For this review, use the dimensioned drawing (mm, ordinates from the lowest corner) and the shaded views. A direction names the side the tool comes from. Coordinates: 2 decimals unless noted, no trailing zeros. Loops run counter-clockwise (first coordinate to the right, second up) from the corner with the lowest first, then second, coordinate; pieces in that order, holes last. Notation, with made-up numbers: M 8,44 L 46,44 A13 cw 46,55 Z; hole C -20,70 d2. An arc over 180 degrees is marked long. One line per item, written item: value.
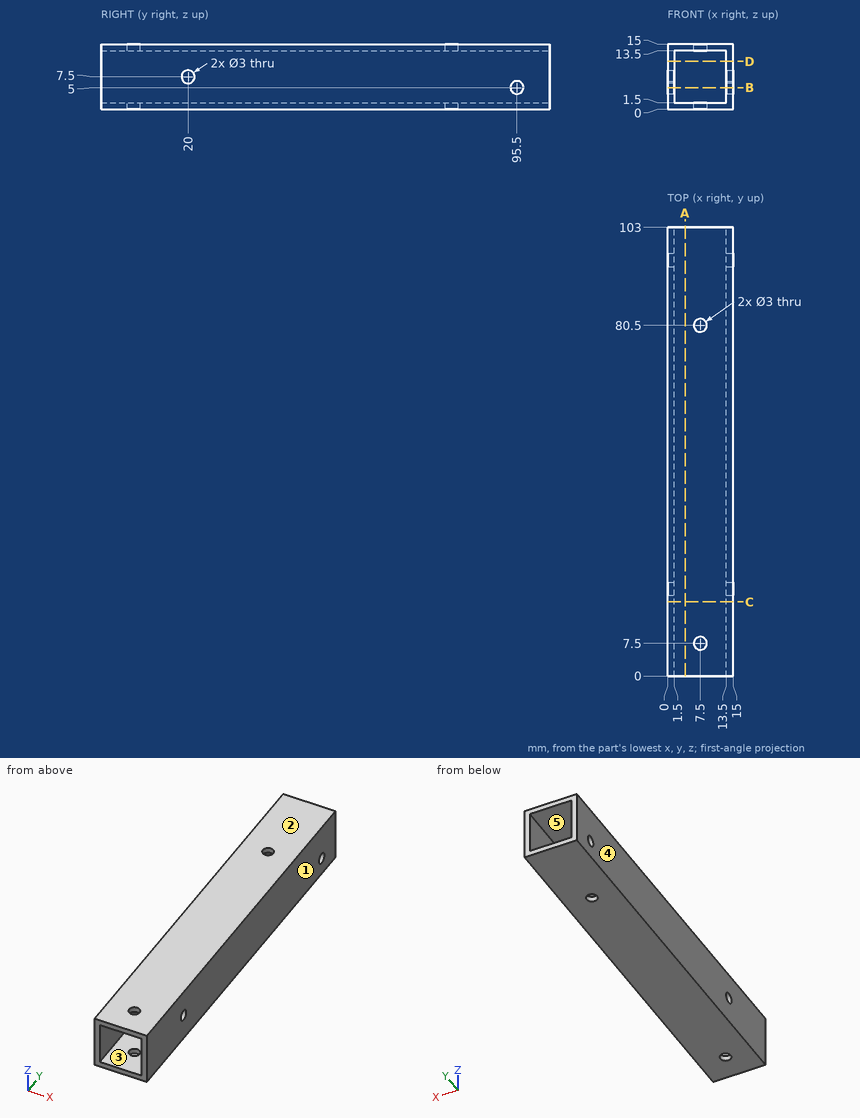
(1) To check wall thickness, follow line 1 along Y through (x, z) = (7.5, 14.1); line 2 along X through (y, z) = (46, 3); line 3 along Y through (x, z) = (0.45, 5). State the ranges of each line that lie inside material, in increasing order. Write a range as [from, to].
Reply:
line 1: y = [0, 6], [9, 79], [82, 103]
line 2: x = [0, 1.5], [13.5, 15]
line 3: y = [0, 94], [97, 103]
(2) We need section C-C on y = 17. State the section outline as (x, z) points.
Reply:
outline: M 0,0 L 15,0 L 15,15 L 0,15 Z; hole M 1.5,1.5 L 13.5,1.5 L 13.5,13.5 L 1.5,13.5 Z
(3) We need section D-D on z = 11. State the section outline as (x, y) points, then the cut area to 3 significant figures.
Reply:
outline: M 0,0 L 1.5,0 L 1.5,103 L 0,103 Z; M 13.5,0 L 15,0 L 15,103 L 13.5,103 Z
area: 309 mm2
(4) Insertion check: pin 1 (5 mm diameter, centred on y = 75, z = 12.5, fed in from -X); pin 2 (2.5 mm diameter, centred on x = 7.5, y = 80.5, fed in from -Z). Each pin has a flat end and moves straight along its axis. Give the tip position at first contact, or say it passes through.
Reply:
pin 1: stops at x = 0
pin 2: passes through
(5) We need section A-A on x = 4. State the section outline as (y, z) points, then the cut area to 3 significant figures.
Reply:
outline: M 0,0 L 103,0 L 103,1.5 L 0,1.5 Z; M 0,13.5 L 103,13.5 L 103,15 L 0,15 Z
area: 309 mm2
(6) Tool access review of the marked faces 4 and 5: name each direction out of +Z, -Z, +X, -X, +Y, -Y from which nothing blocks a thin tool from reaching the whole face with its end or side.
Reply:
face 4: +Z, -Z, -X, +Y, -Y
face 5: +Y, -Y
(7) Mouldability with a two-part tool opening along X and no side actions: class the marked faces 1, 2 and 3 as released by +X, released by -X, zero draft, split by the parting line, or undercut.
Reply:
face 1: released by +X
face 2: zero draft
face 3: undercut
(8) We need section B-B on z = 5. State the section outline as (x, y) points, then the cut area to 3 significant figures.
Reply:
outline: M 0,0 L 1.5,0 L 1.5,94 L 0,94 Z; M 0,97 L 1.5,97 L 1.5,103 L 0,103 Z; M 13.5,0 L 15,0 L 15,94 L 13.5,94 Z; M 13.5,97 L 15,97 L 15,103 L 13.5,103 Z
area: 300 mm2
